Verification items for the finished model (mm, model axes). A direction names the side the tool comes from. Round coordinates to 2 decimals unless told otherwise and drop trailing zeros. Write each loop counter-clockwise with the first axis right and the second up, starting at its lowest first coordinate (ties: lowest second). Pieces come first, ordered by that corner, then holes. Notation, with made-up numbers: M 14,4 L 25,4 A32 cw 25,31 Z; hole C -22,34.5 d1. An arc over 180 degrees is marked long. One line per question, with ' | ' between items. Start each with the question number.
Q1. Cross-section at D-D (y = 11). Record the boundary of the cut face in (x, z).
Q2. Release check for a two-part mould opening along Z. For faces 3 (the face through (-13, 9.4, 0)), 4 (the face through (-0.13, 13.76, 8.91)), 5 (the face through (13.64, 4.77, -13.69)) record: released by +Z, released by -Z, zero draft, split by the parting line, or undercut.
Q3. Cross-section at C-C (y = 15.5). Record the boundary of the cut face in (x, z).
Q4. Tool access check on faces 1 (the face through (-8.91, 13.76, 0.13)), 2 (the face through (-0.161, 4.634, 14.567)). Record the directions out of +Z, -Z, +X, -X, +Y, -Y that give a thin tool (end or side, any length) a straight path to the whole face; none if there is none.
Q5. Cross-section at B-B (x = 2.25). Record the boundary of the cut face in (y, z).
Q6. Cross-section at A-A (z = 7.75). Record the boundary of the cut face in (x, y), then the cut area to 3 significant figures.
Q7. Thickness scan on line 1 along Y through (x, z) = (-7.75, -0.75); line 2 along Y through (x, z) = (-6.25, 12.25); line 3 along X through (y, z) = (15, -0.25). Record the ranges inside material, lowest first. Write a range as from..to.
Q8. Gauge pin test, flat ends, axial feed: pin 1 (13.5 mm diameter, centred on x = 1.5, z = 0, fed in from +Y); pin 2 (6 mm diameter, centred on y = 5, z = -9, fed in from +X); pin 3 (10 mm diameter, centred on y = 21.5, z = -1.5, fed in from -X). Record the tip position at first contact, or that the pin passes through.
from build123d import *

# Parameters (mm, degrees)
SKETCH1_W           = 27
SKETCH1_H           = 27
BOSS_EXTRUDE1_DEPTH = 25
SKETCH2_W           = 27
SKETCH2_H           = 27
SKETCH2_W_2         = 22.6
SKETCH2_H_2         = 22.6
CUT_EXTRUDE1_DEPTH  = 15.6
SKETCH3_W           = 19
SKETCH3_H           = 19
CUT_EXTRUDE2_DEPTH  = 22.8
FILLET1_R           = 0.5
FILLET2_R           = 2
DRAFT12_ANGLE       = 3


with BuildPart() as part:
    # Sketch1 → Boss-Extrude1 (new body)
    with BuildSketch(Plane(origin=(0, 0, 0), x_dir=(1, 0, 0), z_dir=(0, 1, 0))):
        Rectangle(SKETCH1_W, SKETCH1_H)
    extrude(amount=BOSS_EXTRUDE1_DEPTH)

    # Sketch2 → Cut-Extrude1 (cut)
    with BuildSketch(Plane(origin=(0, 25, 0), x_dir=(1, 0, 0), z_dir=(0, 1, 0))):
        Rectangle(SKETCH2_W, SKETCH2_H)
        Rectangle(SKETCH2_W_2, SKETCH2_H_2, mode=Mode.SUBTRACT)
    extrude(amount=-CUT_EXTRUDE1_DEPTH, mode=Mode.SUBTRACT)

    # Sketch3 → Cut-Extrude2 (cut)
    with BuildSketch(Plane(origin=(0, 25, 0), x_dir=(1, 0, 0), z_dir=(0, 1, 0))):
        Rectangle(SKETCH3_W, SKETCH3_H)
    extrude(amount=-CUT_EXTRUDE2_DEPTH, mode=Mode.SUBTRACT)

    # Fillet1
    fillet1_edges = [part.edges().sort_by_distance(p)[0] for p in [
        (-11.3, 17.2, 11.3),
        (-11.3, 17.2, -11.3),
        (11.3, 17.2, -11.3),
        (11.3, 17.2, 11.3),
    ]]
    fillet(fillet1_edges, radius=FILLET1_R)

    # Fillet2
    fillet2_edges = [part.edges().sort_by_distance(p)[0] for p in [
        (-13.5, 4.7, -13.5),
        (13.5, 4.7, -13.5),
        (13.5, 4.7, 13.5),
        (-13.5, 4.7, 13.5),
    ]]
    fillet(fillet2_edges, radius=FILLET2_R)

    # Draft12
    draft12_faces = [part.faces().sort_by_distance(p)[0] for p in [
        (13.5, 4.7, 0),
        (9.5, 13.6, 0),
        (0, 13.6, 9.5),
        (-9.5, 13.6, 0),
        (0, 13.6, -9.5),
        (-11.153553391, 17.2, -11.153553391),
        (-12.914213562, 4.7, -12.914213562),
        (-13.5, 4.7, 0),
        (-11.3, 17.2, 0),
        (-11.153553391, 17.2, 11.153553391),
        (-12.914213562, 4.7, 12.914213562),
        (0, 4.7, 13.5),
        (12.914213562, 4.7, 12.914213562),
        (11.153553391, 17.2, 11.153553391),
        (0, 17.2, 11.3),
        (11.3, 17.2, 0),
        (11.153553391, 17.2, -11.153553391),
        (0, 17.2, -11.3),
        (0, 4.7, -13.5),
        (12.914213562, 4.7, -12.914213562),
    ]]
    draft(draft12_faces, Plane.ZX.offset(25), DRAFT12_ANGLE)


solid = part.part
Determined:
1) outline: M -12.03,-10.8 A1.23 ccw -10.8,-12.03 L 10.8,-12.03 A1.23 ccw 12.03,-10.8 L 12.03,10.8 A1.23 ccw 10.8,12.03 L -10.8,12.03 A1.23 ccw -12.03,10.8 Z; hole M -8.77,-8.77 L 8.77,-8.77 L 8.77,8.77 L -8.77,8.77 Z
2) face 3: zero draft | face 4: undercut | face 5: released by -Z
3) outline: M -11.8,-10.8 A1 ccw -10.8,-11.8 L 10.8,-11.8 A1 ccw 11.8,-10.8 L 11.8,10.8 A1 ccw 10.8,11.8 L -10.8,11.8 A1 ccw -11.8,10.8 Z; hole M -9,-9 L 9,-9 L 9,9 L -9,9 Z
4) face 1: +Y | face 2: +Z, +X, -X, +Y
5) outline: M 0,-14.81 L 9.4,-14.32 L 9.4,-12.12 L 25,-11.3 L 25,-9.5 L 2.2,-8.31 L 2.2,8.31 L 25,9.5 L 25,11.3 L 9.4,12.12 L 9.4,14.32 L 0,14.81 Z
6) outline: M -14.81,0 L 14.81,0 L 14.32,9.4 L 12.12,9.4 L 11.3,25 L 9.5,25 L 8.31,2.2 L -8.31,2.2 L -9.5,25 L -11.3,25 L -12.12,9.4 L -14.32,9.4 Z | area: 233 mm²
7) line 1: y = 0..2.2 | line 2: y = 0..9.4 | line 3: x = -11.82..-8.98, 8.98..11.82
8) pin 1: stops at y = 2.2 | pin 2: stops at x = 14.71 | pin 3: stops at x = -11.75
